Source: CAD feature listing. Evaluate the final solid. Frame: model axes, mm. A direction names the side the tool comes from. Give positions to 0.01 mm unless a question says otherwise; leave off trailing zeros. Loops run counter-clockwise (first coordinate to the right, second up) from the corner with the lowest first, then second, coordinate; pieces in that order, holes last. Notation, with made-up numbers: (70.25, -21) -> (99.25, -21) arc R20 cw to (99.25, -17) -> close; hole circle Ø8 at (45, 62). An arc over 180 degrees is marked (long way). Answer as a JSON object with one key per item and string values. Group by question number.
from build123d import *

# Parameters (mm, degrees)
F1_DEPTH = 60
F4_DEPTH = 20.001
F5_R     = 8
F6_DEPTH = 120.001


with BuildPart() as f1:
    # F0 (on Front) → F1 (new body)
    with BuildSketch(Plane.XZ):
        Polygon((-40, -28.375002), (-80, -28.375002), (-80, -48.375002), (80, -48.375002), (80, -28.375002), (40, -28.375002), (0, -28.375002), align=None)
        with BuildLine():
            Line((-40, 11.624998), (-40, -28.375002))
            Line((-40, -28.375002), (0, -28.375002))
            Line((0, -28.375002), (0, -18.375002))
            ThreePointArc((0, -18.375002), (-21.213203, -9.588205), (-30, 11.624998))
            Line((-30, 11.624998), (-40, 11.624998))
        make_face()
        with BuildLine():
            Line((0, -18.375002), (0, -28.375002))
            Line((0, -28.375002), (40, -28.375002))
            Line((40, -28.375002), (40, 11.624998))
            Line((40, 11.624998), (30, 11.624998))
            ThreePointArc((30, 11.624998), (21.213203, -9.588205), (0, -18.375002))
        make_face()
    extrude(amount=F1_DEPTH)

    # F3 (on face) → F4 (cut, through all)
    with BuildSketch(Plane.XY.offset(-28.375002)):
        with BuildLine():
            ThreePointArc((-60.433533, -12.584707), (-66.433533, -6.584707), (-72.433533, -12.584707))
            Line((-72.433533, -12.584707), (-72.433533, -46.584707))
            ThreePointArc((-72.433533, -46.584707), (-66.433533, -52.584707), (-60.433533, -46.584707))
            Line((-60.433533, -46.584707), (-60.433533, -12.584707))
        make_face()
        with BuildLine():
            ThreePointArc((62.259354, -50.032701), (68.259354, -56.032701), (74.259354, -50.032701))
            Line((74.259354, -50.032701), (74.259354, -16.032701))
            ThreePointArc((74.259354, -16.032701), (68.259354, -10.032701), (62.259354, -16.032701))
            Line((62.259354, -16.032701), (62.259354, -50.032701))
        make_face()
    extrude(amount=-F4_DEPTH, mode=Mode.SUBTRACT)

    # F5 (on face) → F6 (cut, through all)
    with BuildSketch(Plane.YZ.offset(40)):
        with Locations((-29.667338, -7.530242)):
            Circle(F5_R)
    extrude(amount=-F6_DEPTH, mode=Mode.SUBTRACT)


solid = f1.part
(1) First-contact query: pin 1 (10 mm diameter, centred on y = -50.5, z = 0.5, fed in from -X); pin 2 (20 mm diameter, centred on x = 56.5, y = -18.5, fed in from +Z) (3 decimals). Flat tips, straight axial feed; report the tip coordinate or a pass-through.
(2) Section query D-D on y = -32. Return the cut outline in (x, z) (3 decimals), plus the area to 3 significant figures.
(3) Access query for faces 5 (the face through (-40, -23, -13)), 6 (the face through (-66.302, -6.586, -38.235)), 7 (the face through (40, -36, -13)). Directions: +Z, -Z, +X, -X, +Y, -Y. A direction counts if a zero-diameter tool reaches every point of the face in a straight line with its end or side. Return the directions, or none.
(4) Material intervals for line 1 (X direction, y = -40, z = -29.5); line 2 (X direction, y = -48.5, z = -34); line 3 (X direction, y = -38.5, z = -27), sorted ascending. Write a range as from..to.
(5) Section query B-B on x = -68. Return the cut outline in (y, z) (3 decimals), plus the area to 3 significant figures.
(6) Section query C-C on z = -42. Return the cut outline in (x, y).
(7) Section query A-A on y = -42. Return the cut outline in (x, z) (3 decimals), plus the area to 3 significant figures.
(8) Mould query, pull axis Y, two halves, no side actions, for faces 1 (the face through (62.259, -33, -38)), 2 (the face through (-80, -30, -38)), 3 (the face through (-1, -60, -25)), 4 (the face through (68.391, -10.034, -38.235)). Classes: pulls with the +Y half, pulls with the -Y half, needs draft (parallel to the pull), parting line crosses it, or undercut.
Result:
{
 "1": {"pin 1": "x = -40", "pin 2": "z = -28.375"},
 "2": {"outline": "(-80, -48.375) -> (-72.434, -48.375) -> (-72.434, -28.375) -> (-80, -28.375) -> close; (-60.434, -48.375) -> (62.259, -48.375) -> (62.259, -28.375) -> (40, -28.375) -> (40, -15.183) -> (13.467, -15.183) arc R30 cw to (0, -18.375) arc R30 cw to (-13.467, -15.183) -> (-40, -15.183) -> (-40, -28.375) -> (-60.434, -28.375) -> close; (-40, 0.122) -> (-27.707, 0.122) arc R30 cw to (-30, 11.625) -> (-40, 11.625) -> close; (27.707, 0.122) -> (40, 0.122) -> (40, 11.625) -> (30, 11.625) arc R30 cw to start; (74.259, -48.375) -> (80, -48.375) -> (80, -28.375) -> (74.259, -28.375) -> close", "area": "3,960 mm²"},
 "3": {"face 5": "+Z, -X, +Y, -Y", "face 6": "+Z, -Z", "face 7": "+Z, +X, +Y, -Y"},
 "4": {"line 1": "-80..-72.43, -60.43..62.26, 74.26..80", "line 2": "-80..-72.12, -60.75..62.26, 74.26..80", "line 3": "-40..40"},
 "5": {"outline": "(-60, -48.375) -> (-52.377, -48.375) -> (-52.377, -28.375) -> (-60, -28.375) -> close; (-6.793, -48.375) -> (0, -48.375) -> (0, -28.375) -> (-6.793, -28.375) -> close", "area": "288 mm²"},
 "6": {"outline": "(-80, -60) -> (80, -60) -> (80, 0) -> (-80, 0) -> close; hole (-72.43, -46.58) arc R6 ccw to (-60.43, -46.58) -> (-60.43, -12.58) arc R6 ccw to (-72.43, -12.58) -> close; hole (62.26, -50.03) arc R6 ccw to (74.26, -50.03) -> (74.26, -16.03) arc R6 ccw to (62.26, -16.03) -> close"},
 "7": {"outline": "(-80, -48.375) -> (-72.434, -48.375) -> (-72.434, -28.375) -> (-80, -28.375) -> close; (-60.434, -48.375) -> (62.259, -48.375) -> (62.259, -28.375) -> (40, -28.375) -> (40, 11.625) -> (30, 11.625) arc R30 cw to (0, -18.375) arc R30 cw to (-30, 11.625) -> (-40, 11.625) -> (-40, -28.375) -> (-60.434, -28.375) -> close; (74.259, -48.375) -> (80, -48.375) -> (80, -28.375) -> (74.259, -28.375) -> close", "area": "4,510 mm²"},
 "8": {"face 1": "undercut", "face 2": "needs draft", "face 3": "pulls with the -Y half", "face 4": "undercut"}
}
